Print and shaded views of the part. All mm, measured from the part's lowest x, y and z. A direction names the side the tool comes from. Coordinates: 2 decimals unless noted, no trailing zeros. Loops run counter-clockwise (first coordinate to the right, second up) from the corner with the lowest first, then second, coordinate; pieces in that order, holes last. Notation, with made-up numbers: M 52.25,-20.5 L 61.25,-20.5 A25 ccw 61.25,18.5 Z; hole C -39.5,-3.5 d4. An arc over 180 degrees is marked long. Answer as CSV lines item,"result". Start each with the question number.
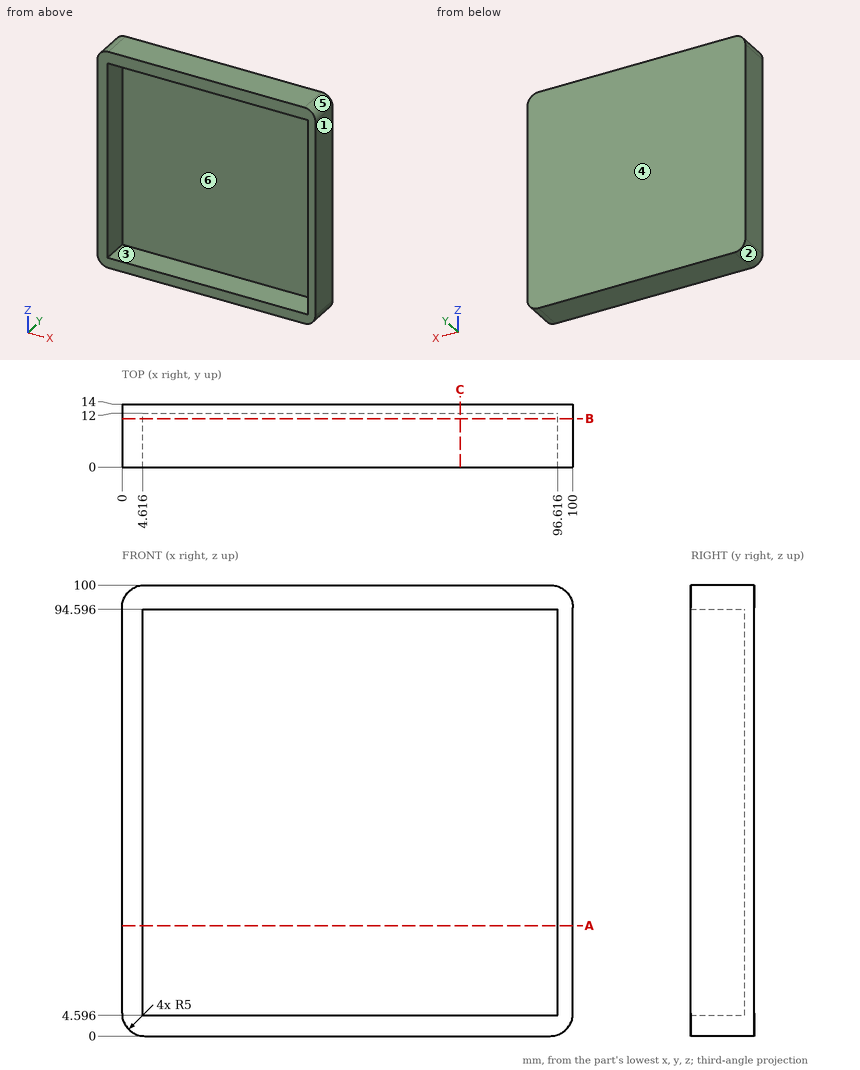
Q1. Flat gauge pin, fed straight in: P1, Ø3.5, axis at y = 4, z = 30, coming from the -X side. Where does the tip first touch, or does it go through?
Q2. Slice it at B-B, the plane y = 10.75. Write the cut outline in (x, z).
Q3. Wall check: L1, parallel to X at y = 8.5, z = 77.5; L2, parallel to Z at x = 15, y = 10; L3, parallel to Y at x = 66, z = 49.5. Give the ranges that are in metal, low to high.
Q4. Two-plate mould, pull along X, no slides. Class the marked faces 1, 2, 3 and 4: +X half, -X half, draft (parallel to the pull), parting line (faces both ways), or undercut.
Q5. Slice it at A-A, the plane z = 24.5. Write the cut outline in (x, y).
Q6. Slice it at C-C, the plane x = 75. Write the cut outline in (y, z).
Q7. Tool access for the marked faces 5 and 6: list every direction of +Z, -Z, +X, -X, +Y, -Y with a clear straight run to the whole face (end or side of a thin tool).
Solved:
1,P1,"stops at x = 0"
2,outline,"M 0,5 A5 ccw 5,0 L 95,0 A5 ccw 100,5 L 100,95 A5 ccw 95,100 L 5,100 A5 ccw 0,95 Z; hole M 4.62,4.6 L 96.62,4.6 L 96.62,94.6 L 4.62,94.6 Z"
3,L1,"x = 0 to 4.62, 96.62 to 100"
3,L2,"z = 0 to 4.6, 94.6 to 100"
3,L3,"y = 12 to 14"
4,face 1,"+X half"
4,face 2,"-X half"
4,face 3,"undercut"
4,face 4,"draft"
5,outline,"M 0,0 L 4.62,0 L 4.62,12 L 96.62,12 L 96.62,0 L 100,0 L 100,14 L 0,14 Z"
6,outline,"M 0,0 L 14,0 L 14,100 L 0,100 L 0,94.6 L 12,94.6 L 12,4.6 L 0,4.6 Z"
7,face 5,"+Z, +X, +Y, -Y"
7,face 6,"-Y"
